```python
from build123d import *

# Parameters (mm, degrees)
F3_D     = 7.9375
F3_DEPTH = 17.4625
F3_TIP   = 2.3846655818
F4_R     = 3.175


with BuildPart() as f1:
    # F0 (on Front) → F1 (revolve)
    with BuildSketch(Plane.XZ):
        with BuildLine():
            add(Edge.make_bspline(
                [(19.852049869, 0), (13.2346999127, 0), (6.6173499563, 0), (0, 0)],
                knots=[0, 0, 0, 0, 0.5, 0.5, 0.5, 0.5], degree=3))
            Line((19.852049869, 0), (22.098, 8.382))
            Line((22.098, 8.382), (25.4, 8.382))
            Line((25.4, 8.382), (24.1662252473, 22.4841099534))
            ThreePointArc((24.1662252473, 22.4841099534), (12.1707524158, 24.6683933927), (0, 25.4))
            Line((0, 25.4), (0, 0))
        make_face()
    revolve(axis=Axis((0, 0, 12.7), (0, 0, -1)))

    # F3
    with Locations(Plane(origin=(0, 0, 0), x_dir=(1, 0, 0), z_dir=(0, 0, -1))):
        with Locations((0, 0)):
            Hole(F3_D / 2, depth=F3_DEPTH)
            with Locations((0, 0, -(F3_DEPTH + F3_TIP / 2))):  # 118° drill point
                Cone(0, F3_D / 2, F3_TIP, mode=Mode.SUBTRACT)

    # F4
    f4_edges = [f1.edges().sort_by_distance(p)[0] for p in [
        (-24.166225, 0, 22.48411),
    ]]
    fillet(f4_edges, radius=F4_R)


solid = f1.part
```
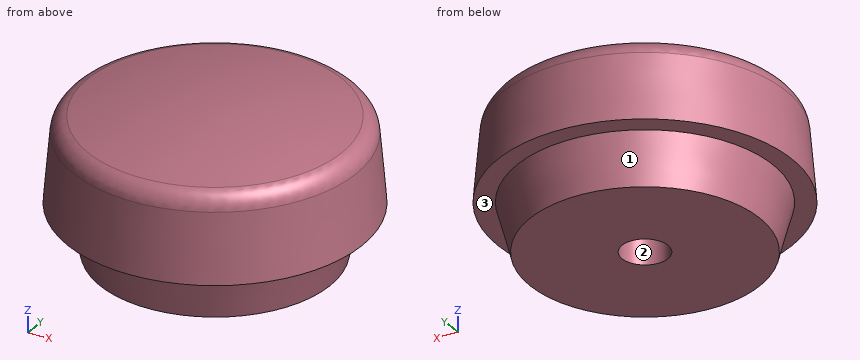
Read the model definition and answer for the solid it produces. Units are mm, in the model's axes. Face numbers are marked on the shaded views. Give positions to 0.01 mm unless a question says otherwise; leave off trailing zeros. Write each loop counter-clockwise with the first axis right and the second up, starting at its lowest first coordinate (ties: lowest second). Pieces come first, ordered by that corner, then holes. Notation, with made-up numbers: (23.25, 62.5) -> (54.25, 62.5) arc R22 cw to (54.25, 90.5) -> close; hole circle Ø1 at (9, 45). An arc over 180 degrees is marked (long way). Answer as a JSON object with one key per item and string values.
1) For a pull along Y with two mould halves and no side action, classify the marked faces 1, 2 and 3 as pulls with the +Y half, pulls with the -Y half, needs draft (parallel to the pull), parting line crosses it, or undercut.
Findings below:
{"face 1": "parting line crosses it", "face 2": "undercut", "face 3": "needs draft"}
2) Flat-ended cylindrical pins translate along their axes: pin 1 Ø4 at (x, y) = (-20, 9.5) entering from +Z; pin 2 Ø3 at (y, z) = (-5.5, 21) entering from -X; pin 3 Ø5 at (x, y) = (-7, -1) entering from +Z. Find the tip coordinate at first contact, or state that the pin passes through.
Findings below:
{"pin 1": "stops at z = 23.38", "pin 2": "stops at x = -24", "pin 3": "stops at z = 25.3"}
3) Section A-A on z = 9.25 is taken. Write down the section's boundary in (x, y), then the cut area to 3 significant figures.
Findings below:
{"outline": "circle Ø50.65 at (0, 0); hole circle Ø7.94 at (0, 0)", "area": "1,970 mm^2"}
4) Section B-B on z = 14.5 is taken. Write down the section's boundary in (x, y), then the cut area to 3 significant figures.
Findings below:
{"outline": "circle Ø49.73 at (0, 0); hole circle Ø7.94 at (0, 0)", "area": "1,890 mm^2"}
5) Straight lines are drawn through the part: probe 1 along Y at (x, z) = (0, 6.5); probe 2 along Y at (x, z) = (0, 9.75); probe 3 along Y at (x, z) = (9.5, 4.25). For each, find the intervals that lie inside material, in ascending order. Write a range as from..to.
Findings below:
{"probe 1": "y = -21.59..-3.97, 3.97..21.59", "probe 2": "y = -25.28..-3.97, 3.97..25.28", "probe 3": "y = -18.72..18.72"}
